from build123d import *

# Parameters (mm, degrees)
F1_DEPTH = 3
F0_W     = 16
F0_H     = 20
F0_W_2   = 3
F0_H_2   = 15.5
F2_DEPTH = 5
F3_SIZE  = 2


with BuildPart() as f1:
    # F0 (on Top) → F1 (new body)
    with BuildSketch(Plane.XY):
        Polygon((1.5, -7.75), (1.5, 7.75), (-1.5, 7.75), align=None)
        Polygon((1.5, -7.75), (-1.5, 7.75), (-1.5, -7.75), align=None)
    extrude(amount=F1_DEPTH)

    # F0 (on Top) → F2 (join)
    with BuildSketch(Plane.XY):
        Rectangle(F0_W, F0_H)
        Rectangle(F0_W_2, F0_H_2, mode=Mode.SUBTRACT)
    extrude(amount=F2_DEPTH)

    # F3
    f3_edges = [f1.edges().sort_by_distance(p)[0] for p in [
        (8, 0, 5),
        (-8, 0, 5),
    ]]
    chamfer(f3_edges, length=F3_SIZE)


solid = f1.part
Geometry: final body of the model. Coordinates: model frame, mm. A direction names the side the tool comes from. Give positions to 0.01 mm unless a question says otherwise; leave off trailing zeros. Loops run counter-clockwise (first coordinate to the right, second up) from the corner with the lowest first, then second, coordinate; pieces in that order, holes last. Notation, with made-up numbers: (74, -38.5) - (117, -38.5) arc R6 cw to (117, -32.5) - close; hole circle Ø6 at (38, -10). An arc over 180 degrees is marked (long way). Answer as CSV lines item,"result". Start each with the question number.
1. Section C-C, the plane x = -0.75. Return loops of the section in (y, z).
2. Ray query, L1, parallel to X at y = -6.5, z = 3.75; L2, parallel to X at y = -2.75, z = 4.6; L3, parallel to Z at x = -1.25, y = -2. Return the intervals inside material, ascending.
3. Section B-B, the plane y = -5. Return loops of the section in (x, z).
4. Section A-A, the plane z = 4.2. Return loops of the section in (x, y), plus the area to 4 significant figures.
5. Reachability of faces 1 (the face through (-7, 0, 4)), 2 (the face through (-1.5, 0, 4)) from +Z, -Z, +X, -X, +Y, -Y: full face, straight path, thin tool, end or side. Return the list, or none.
6. Pin query (flat end, axial travel): P1, Ø0.6, axis at y = 1, z = 4.5, coming from the -X side. Return the tip coordinate at first contact, or that it passes through.
7. Draft query along Y for faces 3 (the face through (7, 0, 4)), 4 (the face through (0, -7.75, 4)), 5 (the face through (0, 10, 2)). Return one class per face: released by +Y, released by -Y, zero draft, split by the parting line, or undercut.
Answers:
1,outline,"(-10, 0) - (10, 0) - (10, 5) - (7.75, 5) - (7.75, 3) - (-7.75, 3) - (-7.75, 5) - (-10, 5) - close"
2,L1,"x = -7.25 to -1.5, 1.5 to 7.25"
2,L2,"x = -6.4 to -1.5, 1.5 to 6.4"
2,L3,"z = 0 to 3"
3,outline,"(-8, 0) - (8, 0) - (8, 3) - (6, 5) - (1.5, 5) - (1.5, 3) - (-1.5, 3) - (-1.5, 5) - (-6, 5) - (-8, 3) - close"
4,outline,"(-6.8, -10) - (6.8, -10) - (6.8, 10) - (-6.8, 10) - close; hole (-1.5, -7.75) - (1.5, -7.75) - (1.5, 7.75) - (-1.5, 7.75) - close"
4,area,"225.5 mm2"
5,face 1,"+Z, -X, +Y, -Y"
5,face 2,"+Z"
6,P1,"stops at x = -6.8"
7,face 3,"zero draft"
7,face 4,"undercut"
7,face 5,"released by +Y"
